```python
from build123d import *

# Parameters (mm, degrees)
F1_DEPTH = 8
F2_R     = 4
F4_D     = 10.5


with BuildPart() as f1:
    # F0 (on Front) → F1 (new body)
    with BuildSketch(Plane.XZ):
        Polygon((140, 0), (0, 0), (0, -275), (100, -275), (100, -300), (140, -300), align=None)
    extrude(amount=F1_DEPTH)

    # F2
    f2_edges = [f1.edges().sort_by_distance(p)[0] for p in [
        (100, -4, -275),
    ]]
    fillet(f2_edges, radius=F2_R)

    # F4 (through all)
    with Locations(Plane.XZ.offset(8)):
        with Locations((108.6, -270)):
            Hole(F4_D / 2)


solid = f1.part
```
Geometry: final body of the model. Coordinates: model frame, mm. A direction names the side the tool comes from. Give positions to 0.01 mm unless a question says otherwise; leave off trailing zeros. Loops run counter-clockwise (first coordinate to the right, second up) from the corner with the lowest first, then second, coordinate; pieces in that order, holes last. Notation, with made-up numbers: (45, 86) -> (87, 86) arc R34 cw to (87, 122) -> close; hole circle Ø10 at (27, -22). An arc over 180 degrees is marked (long way). Return JSON: item names as keys, results as strings.
Item 1: Section B-B, the plane x = 108.6. Output: boundary loops of the cut face in (y, z).
Filled in:
{"outline": "(-8, -300) -> (0, -300) -> (0, -275.25) -> (-8, -275.25) -> close; (-8, -264.75) -> (0, -264.75) -> (0, 0) -> (-8, 0) -> close"}
Item 2: Section C-C, the plane y = -3. Output: boundary loops of the cut face in (x, z).
Filled in:
{"outline": "(0, -275) -> (96, -275) arc R4 cw to (100, -279) -> (100, -300) -> (140, -300) -> (140, 0) -> (0, 0) -> close; hole circle Ø10.5 at (108.6, -270)"}
Item 3: Access query for faces 5 (the flat face through (69, 0, -148)), 6 (the flat face through (47, -4, -275)). Directions: +Z, -Z, +X, -X, +Y, -Y. A direction counts if a zero-diameter tool reaches every point of the face in a straight line with its end or side. Return the directions, or none.
Filled in:
{"face 5": "+Z, -Z, +X, -X, +Y", "face 6": "-Z, -X, +Y, -Y"}
Item 4: Mould query, pull axis X, two halves, no side actions, for faces 1 (the flat face through (100, -4, -289)), 2 (the cylindrical face through (109.283, -3.944, -264.795)), 3 (the flat face through (140, -4, -152)), 4 (the flat face through (120, -4, -300)). Classes: released by +X, released by -X, zero draft, split by the parting line, or undercut.
Filled in:
{"face 1": "released by -X", "face 2": "undercut", "face 3": "released by +X", "face 4": "zero draft"}
Item 5: Section D-D, the plane x = 38.5. Output: boundary loops of the cut face in (y, z).
Filled in:
{"outline": "(-8, -275) -> (0, -275) -> (0, 0) -> (-8, 0) -> close"}
Item 6: Section A-A, the plane z = -270. Output: boundary loops of the cut face in (x, y).
Filled in:
{"outline": "(0, -8) -> (103.35, -8) -> (103.35, 0) -> (0, 0) -> close; (113.85, -8) -> (140, -8) -> (140, 0) -> (113.85, 0) -> close"}
Item 7: Line query: line 1 (Z direction, x = 109, y = -4.5); line 2 (X direction, y = -3.75, z = -270); line 3 (Z direction, x = 45, y = -7). Output: solid intervals per line, ascending.
Filled in:
{"line 1": "-300 to -275.23, -264.77 to 0", "line 2": "0 to 103.35, 113.85 to 140", "line 3": "-275 to 0"}
Item 8: Pin query (flat end, axial travel): P1, Ø2, axis at x = 48.5, y = -6.5, coming from the -Z side. Return the tip coordinate at first contact, or that it passes through.
Filled in:
{"P1": "z = -275"}
